The model under review builds one solid part; all positions refer to its coordinate system, in mm. Face numbers are marked on the shaded views. A direction names the side the tool comes from. Round coordinates to 2 decimals unless told otherwise and drop trailing zeros. Loops run counter-clockwise (first coordinate to the right, second up) from the corner with the lowest first, then second, coordinate; pieces in that order, holes last. Notation, with made-up numbers: M 88.25,-5 L 146.25,-5 A29 ccw 146.25,34 Z; hole C -19,51 d3. An arc over 180 degrees is marked long. One line per question, with ' | ' between items.
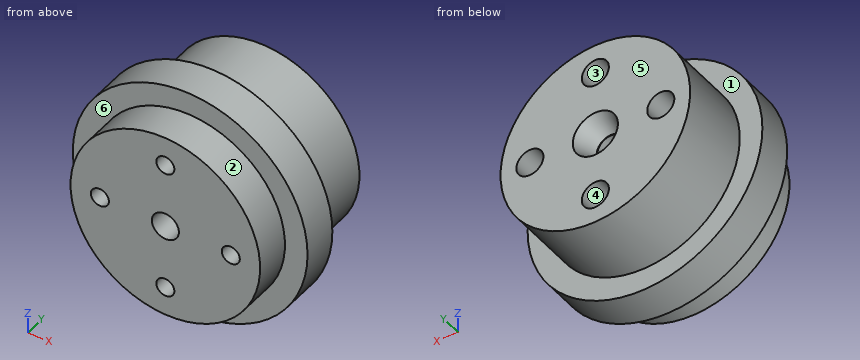
from build123d import *

# Parameters (mm, degrees)
SKETCH1_R                = 10.5
BOSS_EXTRUDE1_DEPTH      = 16
SKETCH2_R                = 1.5
CUT_EXTRUDE1_DEPTH       = 22.828879953
SKETCH3_R                = 2.5
CUT_EXTRUDE2_DEPTH       = 2.5
CUT_EXTRUDE2_DRAFT       = -20.5
BOSS_EXTRUDE2_DEPTH      = 2
BOSS_EXTRUDE2_DEPTH_BACK = 2
SKETCH5_R                = 13
SKETCH7_R                = 1.5
CUT_EXTRUDE3_DEPTH       = 10
SKETCH8_R                = 1
CUT_EXTRUDE4_DEPTH       = 21.928449536
SKETCH9_R                = 1.5
CUT_EXTRUDE5_DEPTH       = 25.372115214


with BuildPart() as part:
    # Sketch1 → Boss-Extrude1 (new body)
    with BuildSketch(Plane(origin=(0, 0, 0), x_dir=(1, 0, 0), z_dir=(0, 1, 0))):
        with Locations(Location((0, 0, 0), (0, 0, 270))):
            Circle(SKETCH1_R)
    extrude(amount=BOSS_EXTRUDE1_DEPTH)

    # Sketch2 → Cut-Extrude1 (cut, through all)
    with BuildSketch(Plane(origin=(0, 16, 0), x_dir=(1, 0, 0), z_dir=(0, 1, 0))):
        with Locations(Location((0, 0, 0), (0, 0, 270))):
            Circle(SKETCH2_R)
    extrude(amount=-CUT_EXTRUDE1_DEPTH, mode=Mode.SUBTRACT)


with BuildPart() as cut_extrude2_tool:
    # Sketch3 → Cut-Extrude2 (with draft: the straight prism first)
    with BuildSketch(Plane(origin=(0, 16, 0), x_dir=(1, 0, 0), z_dir=(0, 1, 0))):
        Circle(SKETCH3_R)
    extrude(amount=-CUT_EXTRUDE2_DEPTH)
    # Cut-Extrude2: the draft: its side faces are tilted about the plane it starts from
    cut_extrude2_sides = [cut_extrude2_tool.faces().sort_by_distance(p)[0] for p in [
        (-2.5, 14.75, 0),
    ]]
    draft(cut_extrude2_sides, Plane(origin=(0, 16, 0), x_dir=(1, 0, 0), z_dir=(0, 1, 0)), CUT_EXTRUDE2_DRAFT)


with BuildPart() as part_1:
    add(part.part)

    # Cut-Extrude2: cut by cut_extrude2_tool
    add(cut_extrude2_tool.part, mode=Mode.SUBTRACT)

    # Sketch5 → Boss-Extrude2 (add, two sides: drawn at the far end of the back side and taken through both)
    with BuildSketch(Plane(origin=(0, 6, 0), x_dir=(-1, 0, 0), z_dir=(0, -1, 0)).offset(-BOSS_EXTRUDE2_DEPTH_BACK)):
        with Locations(Location((0, 0, 0), (0, 0, 90))):
            Circle(SKETCH5_R)
    extrude(amount=BOSS_EXTRUDE2_DEPTH + BOSS_EXTRUDE2_DEPTH_BACK)

    # Sketch7 → Cut-Extrude3 (cut)
    with BuildSketch(Plane(origin=(0, 16, 0), x_dir=(1, 0, 0), z_dir=(0, 1, 0))):
        with Locations(Location((0, 7.25, 0), (0, 0, 270))):
            Circle(SKETCH7_R)
        with Locations(Location((7.25, 0, 0), (0, 0, 270))):
            Circle(SKETCH7_R)
        with Locations(Location((0, -7.25, 0), (0, 0, 270))):
            Circle(SKETCH7_R)
        with Locations(Location((-7.25, 0, 0), (0, 0, 270))):
            Circle(SKETCH7_R)
    extrude(amount=-CUT_EXTRUDE3_DEPTH, mode=Mode.SUBTRACT)

    # Sketch8 → Cut-Extrude4 (cut, through all)
    with BuildSketch(Plane(origin=(0, 6, 0), x_dir=(1, 0, 0), z_dir=(0, 1, 0))):
        with Locations(Location((-7.25, 0, 0), (0, 0, 270))):
            Circle(SKETCH8_R)
        with Locations(Location((0, 7.25, 0), (0, 0, 270))):
            Circle(SKETCH8_R)
        with Locations(Location((7.25, 0, 0), (0, 0, 270))):
            Circle(SKETCH8_R)
        with Locations(Location((0, -7.25, 0), (0, 0, 270))):
            Circle(SKETCH8_R)
    extrude(amount=-CUT_EXTRUDE4_DEPTH, mode=Mode.SUBTRACT)

    # Sketch9 → Cut-Extrude5 (cut, through all)
    with BuildSketch(Plane(origin=(0, 16, 0), x_dir=(1, 0, 0), z_dir=(0, 1, 0))):
        with Locations(Location((0, 0, 0), (0, 0, 270))):
            Circle(SKETCH9_R)
    extrude(amount=-CUT_EXTRUDE5_DEPTH, mode=Mode.SUBTRACT)


solid = part_1.part
1) Add section C-C on z = -7.25. State the section outline as (x, y) points.
Output values:
outline: M -10.79,4 L -7.6,4 L -7.6,0 L -1,0 L -1,6 L -1.5,6 L -1.5,16 L -7.6,16 L -7.6,8 L -10.79,8 Z; M 1,0 L 7.6,0 L 7.6,4 L 10.79,4 L 10.79,8 L 7.6,8 L 7.6,16 L 1.5,16 L 1.5,6 L 1,6 Z
2) For line 1 (X direction, y = 11, z = 0); line 2 (X direction, y = 1.9, z = 0); line 3 (Y direction, x = 5.5, z = 9), list the stretches that pass through material, from the lowest coordinate up.
Output values:
line 1: x = -10.5 to -8.75, -5.75 to -1.5, 1.5 to 5.75, 8.75 to 10.5 | line 2: x = -10.5 to -8.25, -6.25 to -1.5, 1.5 to 6.25, 8.25 to 10.5 | line 3: y = 4 to 8
3) Add section A-A on y = 7.5. State the section outline as (x, z) points, then the cut area to 3 significant figures.
Output values:
outline: C 0,0 d26; hole C -7.25,0 d3; hole C 0,-7.25 d3; hole C 0,0 d3; hole C 0,7.25 d3; hole C 7.25,0 d3 | area: 496 mm²
4) Machinability: for the marked faces 4, 5 and 6, which of the approach directions +Z, -Z, +X, -X, +Y, -Y give a long, thin tool a straight path to every point of the face, cutting with its end or side? Answer none if there is none.
Output values:
face 4: +Y | face 5: +Z, -Z, +X, -X, +Y | face 6: -Y
5) Mouldability with a two-part tool opening along X and no side actions: class the marked faces 1, 2 and 3 as +X half, -X half, draft (parallel to the pull), parting line (faces both ways), or undercut.
Output values:
face 1: draft | face 2: parting line | face 3: undercut
6) Insertion check: P1, Ø2.5, axis at x = -7.25, z = 0, coming from the +Y side; P2, Ø1, axis at x = 1.5, y = 13.5, coming from the +Z side; P3, Ø5, axis at y = 8.5, z = 8.5, coming from the -X side. Each pin has a flat end and moves straight along its axis. Give the tip position at first contact, or say it passes through.
Output values:
P1: stops at y = 6 | P2: stops at z = 10.45 | P3: stops at x = -11.51
7) Add section D-D on x = -7.25. State the section outline as (y, z) points.
Output values:
outline: M 0,-7.6 L 4,-7.6 L 4,-10.79 L 8,-10.79 L 8,-7.6 L 16,-7.6 L 16,-1.5 L 6,-1.5 L 6,-1 L 0,-1 Z; M 0,1 L 6,1 L 6,1.5 L 16,1.5 L 16,7.6 L 8,7.6 L 8,10.79 L 4,10.79 L 4,7.6 L 0,7.6 Z
8) Add section B-B on x = 0. State how many separate pieces and enclosed holes the cut face has, then the cut area to 3 significant figures.
Output values:
separate pieces: 4 | enclosed holes: 0 | area: 221 mm²
